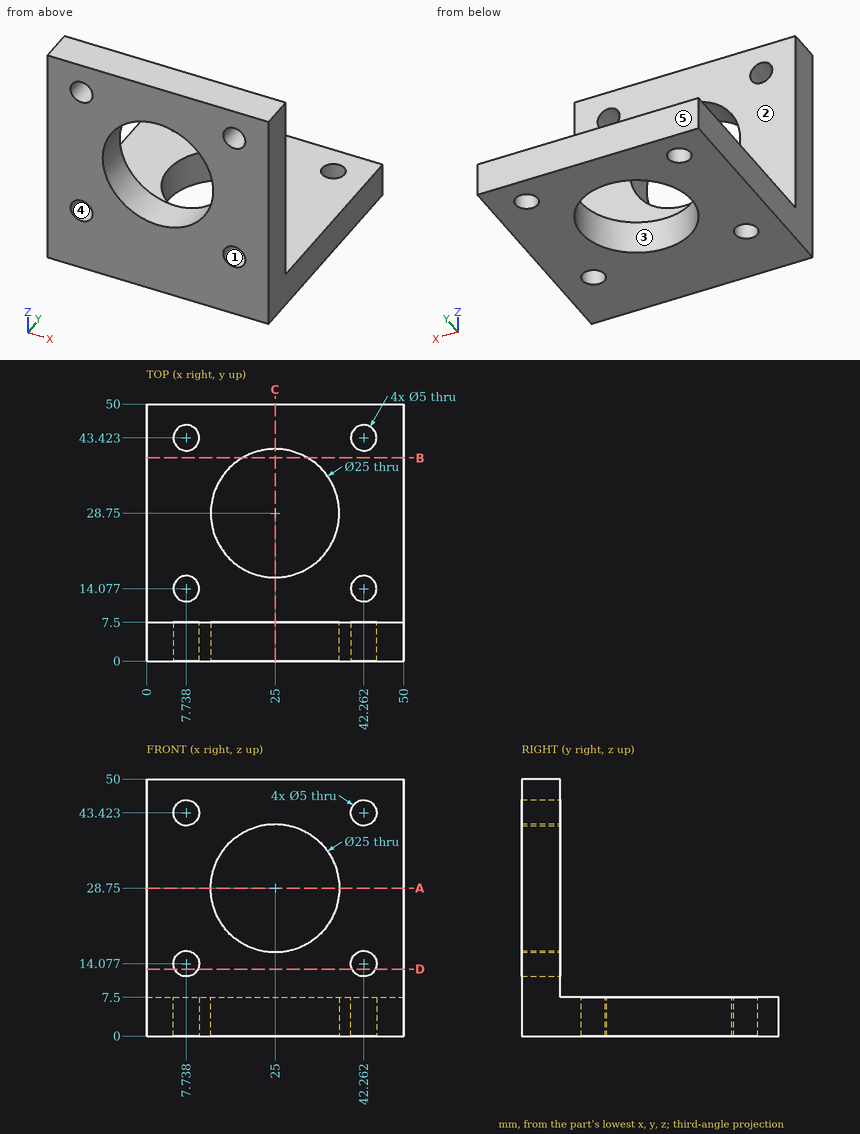
Geometry: see drawing. Coordinates: mm, zero at the bounding-box minimum. A direction names the side the tool comes from. Give positions to 0.01 mm unless a question says otherwise; leave off trailing zeros. Order: outer loops, then holes, each group sorted by start corner. A loop starts at its lowest first (then second) coordinate and runs counter-clockwise, first axis right, second up. Notation, with made-up numbers: (34.5, 57.25) -> (88.5, 57.25) arc R17 cw to (88.5, 65.25) -> close; hole circle Ø7 at (-24.75, 61.25). An arc over 180 degrees is marked (long way). Write item = value, one per line.
Q1. Cut plane D-D, the plane z = 13. Output: boundary loops of the cut face in (x, y).
Data:
outline = (0, 0) -> (5.48, 0) -> (5.48, 7.5) -> (0, 7.5) -> close; (9.99, 0) -> (40.01, 0) -> (40.01, 7.5) -> (9.99, 7.5) -> close; (44.52, 0) -> (50, 0) -> (50, 7.5) -> (44.52, 7.5) -> close
Q2. Cut plane C-C, the plane x = 25. Output: boundary loops of the cut face in (y, z), and give its area (3 significant figures).
Data:
outline = (0, 0) -> (16.25, 0) -> (16.25, 7.5) -> (7.5, 7.5) -> (7.5, 16.25) -> (0, 16.25) -> close; (0, 41.25) -> (7.5, 41.25) -> (7.5, 50) -> (0, 50) -> close; (41.25, 0) -> (50, 0) -> (50, 7.5) -> (41.25, 7.5) -> close
area = 319 mm^2
Q3. Cut plane B-B, the plane y = 39.5. Output: boundary loops of the cut face in (x, z).
Data:
outline = (0, 0) -> (18.62, 0) -> (18.62, 7.5) -> (0, 7.5) -> close; (31.38, 0) -> (50, 0) -> (50, 7.5) -> (31.38, 7.5) -> close
Q4. Cut plane A-A, the plane z = 28.75. Output: boundary loops of the cut face in (x, y).
Data:
outline = (0, 0) -> (12.5, 0) -> (12.5, 7.5) -> (0, 7.5) -> close; (37.5, 0) -> (50, 0) -> (50, 7.5) -> (37.5, 7.5) -> close
Q5. Set-up query: the marked faces 1 and 2. Return all of +Z, -Z, +X, -X, +Y, -Y with unobstructed straight access to the full face (end or side cutting, diameter ignored); none if empty.
Data:
face_1 = +Y, -Y
face_2 = +Z, +X, -X, +Y
Q6. Material intervals for line 1 (Z direction, x = 25, y = 2); line 2 (Y direction, x = 21, z = 12), sorted ascending. Write a range as from..to.
Data:
line_1 = 0..16.25, 41.25..50
line_2 = 0..7.5
Q7. Pull-direction query (Y, two-part tool) for the marked faces 3, 4 and 5; classes: released by +Y, released by -Y, zero draft, split by the parting line, or undercut.
Data:
face_3 = undercut
face_4 = zero draft
face_5 = released by +Y
Q8. Pin query (flat end, axial travel): pin 1 (6 mm diameter, centred on x = 7.74, z = 43.42, fed in from +Y). Return the tip coordinate at first contact, or that it passes through.
Data:
pin_1 = 7.5
